Job drawing, mm, ordinate dimensions from the low corner. One solid piece. A direction names the side the tool comes from. Coordinates: 2 decimals unless noted, no trailing zeros. Loops run counter-clockwise (first coordinate to the right, second up) from the corner with the lowest first, then second, coordinate; pieces in that order, holes last. Notation, with made-up numbers: M 38,56.5 L 84,56.5 A11 ccw 84,77.5 Z; hole C -17.5,54 d11. An arc over 180 degrees is marked long. Answer as a JSON object with one key per item and string values. Group by question number.
1. Drop flat-ended pins along their axis: pin 1 Ø2 at (x, z) = (16.5, 3) entering from -Y; pin 2 Ø6 at (x, z) = (22, 12.5) entering from +Y; pin 3 Ø1 at (x, z) = (21, 11) entering from -Y; pin 4 Ø9 at (x, y) = (10.5, 12.5) entering from -Z. Give the stop position or say it passes through.
2. Saw through at C-C on z = 24. Write the cut outline in (x, y) (3 decimals).
3. Saw through at A-A on y = 12.5. Write the cut outline in (x, z).
4. Saw through at D-D on z = 14. Write the cut outline in (x, y) (3 decimals), then the cut area to 3 significant figures.
5. Mould opens along X. For the marked faces 3, 4 and 5 say: released by +X, released by -X, zero draft, split by the parting line, or undercut.
6. Drill centre lines: L1, parallel to X at y = 12.5, z = 0.8; L2, parallel to Z at x = 10.5, y = 14.75; L3, parallel to Y at x = 5.25, z = 7. Where is each one in solid material? Low to high.
7. 3-axis set-ups, long thin cutter, end or side, ignore diameter. For the marked faces 1 and 2: which of +Z, -Z, +X, -X, +Y, -Y reach the whole face in a straight line?
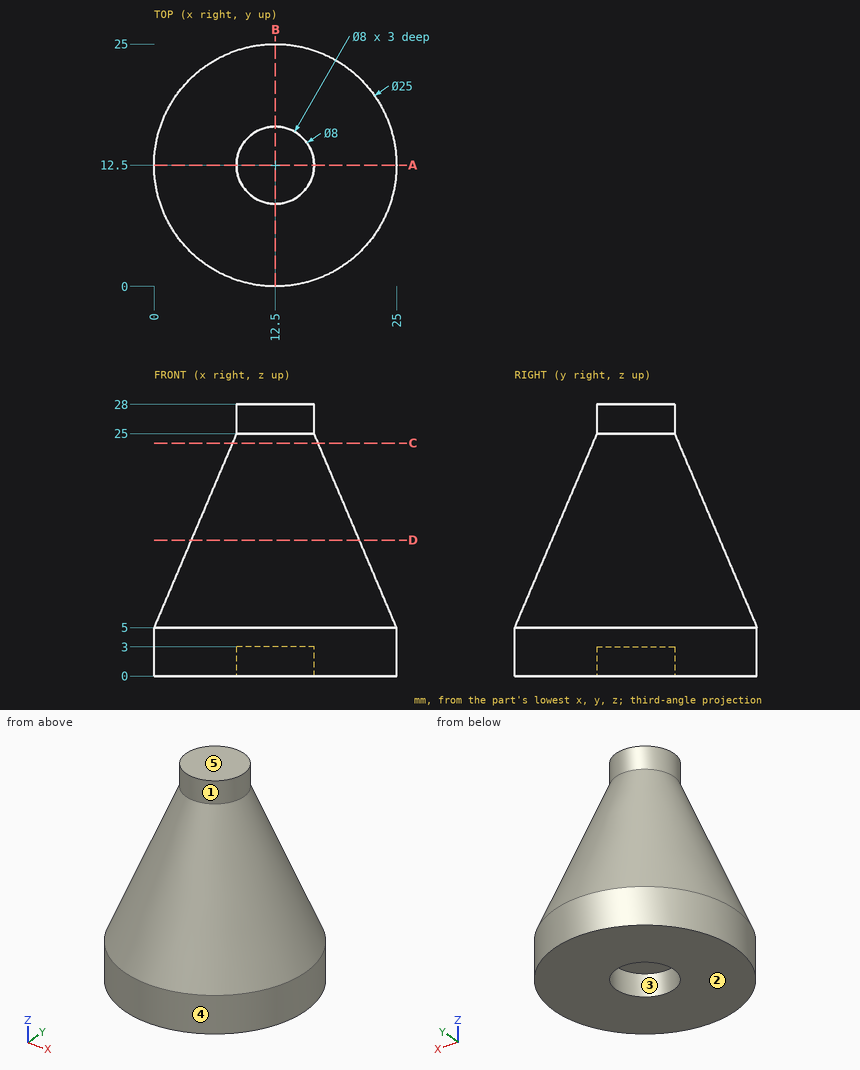
Outcome:
{
 "1": {"pin 1": "stops at y = 0.37", "pin 2": "stops at y = 19.67", "pin 3": "stops at y = 6.5", "pin 4": "stops at z = 0"},
 "2": {"outline": "C 12.5,12.5 d8.85"},
 "3": {"outline": "M 0,0 L 8.5,0 L 8.5,3 L 16.5,3 L 16.5,0 L 25,0 L 25,5 L 16.5,25 L 16.5,28 L 8.5,28 L 8.5,25 L 0,5 Z"},
 "4": {"outline": "C 12.5,12.5 d17.35", "area": "236 mm²"},
 "5": {"face 3": "undercut", "face 4": "split by the parting line", "face 5": "zero draft"},
 "6": {"L1": "x = 0 to 8.5, 16.5 to 25", "L2": "z = 3 to 28", "L3": "y = 3.38 to 21.62"},
 "7": {"face 1": "+Z", "face 2": "-Z, +X, -X, +Y, -Y"}
}
